Verification items for the finished model (mm, model axes). Face numbers are marked on the shaded views. A direction names the side the tool comes from. Coordinates: 2 decimals unless noted, no trailing zeros. Loops run counter-clockwise (first coordinate to the right, second up) from the corner with the lowest first, then second, coordinate; pieces in that order, holes last. Notation, with made-up numbers: (-9.75, 43) -> (15.25, 43) arc R20 cw to (15.25, 75) -> close; hole circle Ø1 at (18.5, 61). An arc over 180 degrees is marked (long way). Write item = value, one per line.
```python
from build123d import *

# Parameters (mm, degrees)
BOSS_EXTRUDE1_DEPTH = 67.55
SKETCH2_W           = 40
SKETCH2_H           = 40
BOSS_EXTRUDE2_DEPTH = 10


with BuildPart() as part:
    # Sketch1 → Boss-Extrude1 (new body)
    with BuildSketch(Plane(origin=(0, 75.994571645, 0), x_dir=(1, 0, 0), z_dir=(0, 1, 0))):
        with BuildLine():
            Line((-75.17747299, -15.039868045), (-60.22747299, -15.039868045))
            Line((-60.22747299, -15.039868045), (-60.22747299, -12.039868045))
            Line((-60.22747299, -12.039868045), (-65.17747299, -12.039868045))
            Line((-65.17747299, -12.039868045), (-65.17747299, -12.539868045))
            Line((-65.17747299, -12.539868045), (-67.763259428, -12.539868045))
            ThreePointArc((-67.763259428, -12.539868045), (-68.68713896, -11.922551477), (-68.470366209, -10.832761264))
            Line((-68.470366209, -10.832761264), (-60.67747299, -3.039868045))
            Line((-60.67747299, -3.039868045), (-49.67747299, -3.039868045))
            Line((-49.67747299, -3.039868045), (-41.884579771, -10.832761264))
            ThreePointArc((-41.884579771, -10.832761264), (-41.66780702, -11.922551477), (-42.591686553, -12.539868045))
            Line((-42.591686553, -12.539868045), (-45.17747299, -12.539868045))
            Line((-45.17747299, -12.539868045), (-45.17747299, -12.039868045))
            Line((-45.17747299, -12.039868045), (-50.12747299, -12.039868045))
            Line((-50.12747299, -12.039868045), (-50.12747299, -15.039868045))
            Line((-50.12747299, -15.039868045), (-35.17747299, -15.039868045))
            Line((-35.17747299, -15.039868045), (-35.17747299, -0.089868045))
            Line((-35.17747299, -0.089868045), (-38.17747299, -0.089868045))
            Line((-38.17747299, -0.089868045), (-38.17747299, -5.039868045))
            Line((-38.17747299, -5.039868045), (-37.67747299, -5.039868045))
            Line((-37.67747299, -5.039868045), (-37.67747299, -7.625654482))
            ThreePointArc((-37.67747299, -7.625654482), (-38.294789558, -8.549534015), (-39.384579771, -8.332761264))
            Line((-39.384579771, -8.332761264), (-47.17747299, -0.539868045))
            Line((-47.17747299, -0.539868045), (-47.17747299, 10.460131955))
            Line((-47.17747299, 10.460131955), (-39.384579771, 18.253025174))
            ThreePointArc((-39.384579771, 18.253025174), (-38.294789558, 18.469797925), (-37.67747299, 17.545918393))
            Line((-37.67747299, 17.545918393), (-37.67747299, 14.960131955))
            Line((-37.67747299, 14.960131955), (-38.17747299, 14.960131955))
            Line((-38.17747299, 14.960131955), (-38.17747299, 10.010131955))
            Line((-38.17747299, 10.010131955), (-35.17747299, 10.010131955))
            Line((-35.17747299, 10.010131955), (-35.17747299, 24.960131955))
            Line((-35.17747299, 24.960131955), (-50.12747299, 24.960131955))
            Line((-50.12747299, 24.960131955), (-50.12747299, 21.960131955))
            Line((-50.12747299, 21.960131955), (-45.17747299, 21.960131955))
            Line((-45.17747299, 21.960131955), (-45.17747299, 22.460131955))
            Line((-45.17747299, 22.460131955), (-42.591686553, 22.460131955))
            ThreePointArc((-42.591686553, 22.460131955), (-41.66780702, 21.842815388), (-41.884579771, 20.753025174))
            Line((-41.884579771, 20.753025174), (-49.67747299, 12.960131955))
            Line((-49.67747299, 12.960131955), (-60.67747299, 12.960131955))
            Line((-60.67747299, 12.960131955), (-68.470366209, 20.753025174))
            ThreePointArc((-68.470366209, 20.753025174), (-68.68713896, 21.842815388), (-67.763259428, 22.460131955))
            Line((-67.763259428, 22.460131955), (-65.17747299, 22.460131955))
            Line((-65.17747299, 22.460131955), (-65.17747299, 21.960131955))
            Line((-65.17747299, 21.960131955), (-60.22747299, 21.960131955))
            Line((-60.22747299, 21.960131955), (-60.22747299, 24.960131955))
            Line((-60.22747299, 24.960131955), (-75.17747299, 24.960131955))
            Line((-75.17747299, 24.960131955), (-75.17747299, 10.010131955))
            Line((-75.17747299, 10.010131955), (-72.17747299, 10.010131955))
            Line((-72.17747299, 10.010131955), (-72.17747299, 14.960131955))
            Line((-72.17747299, 14.960131955), (-72.67747299, 14.960131955))
            Line((-72.67747299, 14.960131955), (-72.67747299, 17.545918393))
            ThreePointArc((-72.67747299, 17.545918393), (-72.060156423, 18.469797925), (-70.970366209, 18.253025174))
            Line((-70.970366209, 18.253025174), (-63.17747299, 10.460131955))
            Line((-63.17747299, 10.460131955), (-63.17747299, -0.539868045))
            Line((-63.17747299, -0.539868045), (-70.970366209, -8.332761264))
            ThreePointArc((-70.970366209, -8.332761264), (-72.060156423, -8.549534015), (-72.67747299, -7.625654482))
            Line((-72.67747299, -7.625654482), (-72.67747299, -5.039868045))
            Line((-72.67747299, -5.039868045), (-72.17747299, -5.039868045))
            Line((-72.17747299, -5.039868045), (-72.17747299, -0.089868045))
            Line((-72.17747299, -0.089868045), (-75.17747299, -0.089868045))
            Line((-75.17747299, -0.089868045), (-75.17747299, -15.039868045))
        make_face()
    extrude(amount=-BOSS_EXTRUDE1_DEPTH)

    # Sketch2 → Boss-Extrude2 (add)
    with BuildSketch(Plane(origin=(0, 75.994571645, 0), x_dir=(1, 0, 0), z_dir=(0, 1, 0))):
        with Locations((-55.17747299, 4.960131955)):
            Rectangle(SKETCH2_W, SKETCH2_H)
    extrude(amount=BOSS_EXTRUDE2_DEPTH)


solid = part.part
```
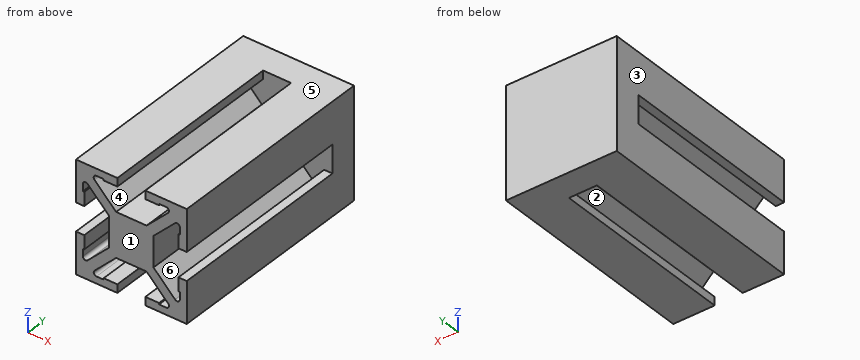
1) Depth check by flat-ended pin: pin 1 Ø3.5 at (x, z) = (-60.5, 7.5) entering from -Y; pin 2 Ø9 at (y, z) = (52, -4.5) entering from +X; pin 3 Ø5.5 at (x, y) = (-53.5, 33.5) entering from -Z. Enter the tip coordinate at first touch or a pass-through.
Ans:
pin_1 = 75.99
pin_2 = -47.18
pin_3 = -12.96
2) Release check for a two-part mould opening along X. For the marked faces 3, 4, 5 and 6 record: pulls with the +X half, pulls with the -X half, needs draft (parallel to the pull), parting line crosses it, or undercut.
Ans:
face_3 = pulls with the -X half
face_4 = undercut
face_5 = needs draft
face_6 = undercut
3) Material ranges on line 1 (Z direction, x = -60.5, y = 63.5); line 2 (Z direction, x = -44.5, y = 58); line 3 (X direction, y = 43, z = -13.5), recorded low to high.
Ans:
line_1 = -24.96 to -21.96, -12.96 to 3.04, 12.04 to 15.04
line_2 = -24.96 to -22.46, -18.14 to -13.14, 3.22 to 8.22, 12.54 to 15.04
line_3 = -75.18 to -72.18, -66.22 to -61.22, -49.14 to -44.14, -38.18 to -35.18
4) Tool access check on the marked faces 1 and 2. Record the directions out of +Z, -Z, +X, -X, +Y, -Y that give a thin tool (end or side, any length) a straight path to the whole face; none if there is none.
Ans:
face_1 = +Z, -Z, +X, -X, -Y
face_2 = -Y
5) Sectioned sample at A-A, the plane x = -57. Record the cut outline in (y, z).
Ans:
outline = (8.44, -12.96) -> (75.99, -12.96) -> (75.99, -24.96) -> (85.99, -24.96) -> (85.99, 15.04) -> (75.99, 15.04) -> (75.99, 3.04) -> (8.44, 3.04) -> close
